```python
from build123d import *

# Parameters (mm, degrees)
BOSS_EXTRUDE1_DEPTH      = 40
CUT_EXTRUDE1_DEPTH       = 45
CUT_EXTRUDE2_REACH       = 47.222
SKETCH3_W                = 12
SKETCH3_H                = 10
SKETCH4_R                = 2.55
CUT_EXTRUDE3_DEPTH       = 17.5
FILLET4_R                = 2
CUT_EXTRUDE5_START       = -12.324555
SKETCH6_R                = 2.5
CUT_EXTRUDE5_DEPTH       = 9.6
CUT_EXTRUDE6_START       = 6.279445
SKETCH6_3_R              = 2.5
CUT_EXTRUDE6_DEPTH       = 6.604
CUT_EXTRUDE7_START       = -14.986
CUT_EXTRUDE7_DEPTH       = 14.986
CUT_EXTRUDE14_DEPTH      = 10
CUT_EXTRUDE14_DEPTH_BACK = 20
FILLET3_R                = 1
CUT_EXTRUDE17_DEPTH      = 9
CUT_EXTRUDE17_DEPTH_BACK = 31
SKETCH19_W               = 34.391960709
SKETCH19_H               = 80.468832088
SKETCH20_R               = 3.25
BOSS_EXTRUDE2_DEPTH      = 2
SKETCH21_R               = 1.5
CUT_EXTRUDE18_DEPTH      = 14
CUT_EXTRUDE19_START      = -4
SKETCH22_R               = 2.5
CUT_EXTRUDE19_DEPTH      = 14
CUT_EXTRUDE20_DEPTH      = 14
CUT_EXTRUDE20_DEPTH_BACK = 14


with BuildPart() as part:
    # Sketch1 → Boss-Extrude1 (new body)
    with BuildSketch(Plane(origin=(0, 0, 0), x_dir=(1, 0, 0), z_dir=(0, 1, 0))):
        with BuildLine():
            Line((-6.32455532, 9), (6.32455532, 9))
            ThreePointArc((6.32455532, 9), (11, 0), (6.32455532, -9))
            Line((6.32455532, -9), (-6.32455532, -9))
            ThreePointArc((-6.32455532, -9), (-11, 0), (-6.32455532, 9))
        make_face()
    extrude(amount=BOSS_EXTRUDE1_DEPTH)

    # Sketch2 → Cut-Extrude1 (cut)
    with BuildSketch(Plane.XZ):
        with BuildLine():
            Line((1.5, 5), (-1.5, 5))
            ThreePointArc((-1.5, 5), (0, 6.5), (1.5, 5))
        make_face()
        with BuildLine():
            Line((1.5, -5), (-1.5, -5))
            ThreePointArc((-1.5, -5), (0, -6.5), (1.5, -5))
        make_face()
    extrude(amount=-CUT_EXTRUDE1_DEPTH, mode=Mode.SUBTRACT)

    # Cut-Extrude2: up to this face of the body (flat: up to its plane)
    cut_extrude2_end = Plane(part.part.faces().sort_by_distance((0, 20, 9))[0])
    # Sketch3 → Cut-Extrude2 (cut, up to the picked face)
    with BuildSketch(Plane(origin=(0, 0, -9), x_dir=(-1, 0, 0), z_dir=(0, 0, -1)), mode=Mode.PRIVATE) as cut_extrude2_sk1:
        with Locations((0, 5)):
            Rectangle(SKETCH3_W, SKETCH3_H)
    cut_extrude2_tool1 = split(extrude(cut_extrude2_sk1.sketch, amount=-CUT_EXTRUDE2_REACH, mode=Mode.PRIVATE), bisect_by=cut_extrude2_end, keep=Keep.BOTH, mode=Mode.PRIVATE)
    add(cut_extrude2_tool1.solids().sort_by(Axis((0, 5, -9), (0, 0, 1)))[0], mode=Mode.SUBTRACT)

    # Sketch4 → Cut-Extrude3 (cut, symmetric)
    with BuildSketch(Plane.ZY.offset(-6)):
        with Locations(Location((0, 4.9, 0), (0, 0, 270))):
            Circle(SKETCH4_R)
        with BuildLine():
            Line((-9, 10), (-4.9, 4.9))
            ThreePointArc((-4.9, 4.9), (0, 0), (4.9, 4.9))
            Line((4.9, 4.9), (9, 10))
            Line((9, 10), (12.043777938, -1.930413563))
            Line((12.043777938, -1.930413563), (-10.290438773, -1.930413563))
            Line((-10.290438773, -1.930413563), (-9, 10))
        make_face()
    extrude(amount=CUT_EXTRUDE3_DEPTH, both=True, mode=Mode.SUBTRACT)

    # Fillet4
    fillet4_edges = [part.edges().sort_by_distance(p)[0] for p in [
        (0, 10, 5),
        (0, 10, 6.5),
        (0, 10, -5),
        (0, 10, -6.5),
    ]]
    fillet(fillet4_edges, radius=FILLET4_R)

    # Sketch6 → Cut-Extrude5 (cut)
    with BuildSketch(Plane.ZY.offset(6.32455532).offset(CUT_EXTRUDE5_START)):
        with BuildLine():
            Line((9, 22.232353468), (0, 30))
            ThreePointArc((0, 30), (-3.535533906, 31.464466094), (-5, 35))
            Line((-5, 35), (-6.715621335, 37.134065563))
            ThreePointArc((-6.715621335, 37.134065563), (-7.737273484, 38.043034193), (-9, 38.567933069))
            Line((-9, 38.567933069), (-20.985236203, 70.297327945))
            Line((-20.985236203, 70.297327945), (29.827478779, 37.594689174))
            Line((29.827478779, 37.594689174), (9, 22.232353468))
        make_face()
        with Locations((0, 35)):
            Circle(SKETCH6_R, mode=Mode.SUBTRACT)
    extrude(amount=-CUT_EXTRUDE5_DEPTH, mode=Mode.SUBTRACT)

    # Sketch6<3> → Cut-Extrude6 (cut)
    with BuildSketch(Plane.ZY.offset(6.32455532).offset(CUT_EXTRUDE6_START)):
        with BuildLine():
            Line((9, 22.232353468), (0, 30))
            ThreePointArc((0, 30), (-3.535533906, 31.464466094), (-5, 35))
            Line((-5, 35), (-6.715621335, 37.134065563))
            ThreePointArc((-6.715621335, 37.134065563), (-7.737273484, 38.043034193), (-9, 38.567933069))
            Line((-9, 38.567933069), (-20.985236203, 70.297327945))
            Line((-20.985236203, 70.297327945), (29.827478779, 37.594689174))
            Line((29.827478779, 37.594689174), (9, 22.232353468))
        make_face()
        with Locations((0, 35)):
            Circle(SKETCH6_3_R, mode=Mode.SUBTRACT)
    extrude(amount=-CUT_EXTRUDE6_DEPTH, mode=Mode.SUBTRACT)

    # Sketch7 → Cut-Extrude7 (cut)
    with BuildSketch(Plane(origin=(6, 0, 0), x_dir=(0, 0, -1), z_dir=(1, 0, 0)).offset(CUT_EXTRUDE7_START)):
        with BuildLine():
            Line((5, 35), (6.715621335, 37.134065563))
            ThreePointArc((6.715621335, 37.134065563), (7.737273484, 38.043034193), (9, 38.567933069))
            Line((9, 38.567933069), (17.905522107, 46.18977372))
            Line((17.905522107, 46.18977372), (-20.628346566, 40.15215478))
            Line((-20.628346566, 40.15215478), (-9, 22.232353468))
            Line((-9, 22.232353468), (-5, 25.684640815))
            Line((-5, 25.684640815), (-5, 35))
            ThreePointArc((-5, 35), (0, 40), (5, 35))
        make_face()
    extrude(amount=CUT_EXTRUDE7_DEPTH, mode=Mode.SUBTRACT)

    # Sketch16 → Cut-Extrude14 (cut, two sides: drawn at the far end of the back side and taken through both)
    with BuildSketch(Plane.ZY.offset(6.32455532).offset(-CUT_EXTRUDE14_DEPTH_BACK)):
        Polygon((8.113259987, 8.896981935), (11.550119513, 20.031417135), (18.056002312, 15.695207893), (16.156055326, 2.281594324), align=None)
    extrude(amount=CUT_EXTRUDE14_DEPTH + CUT_EXTRUDE14_DEPTH_BACK, mode=Mode.SUBTRACT)

    # Fillet3
    # the kernel refuses this fillet: 1 mm, written as the material it takes off along each edge
    with BuildSketch(Plane(origin=(5.99999968, 23.184640014, 5), x_dir=(-1, 0, 0), z_dir=(0, 1, 0))) as fillet3_piece_1_section:
        with BuildLine():
            CenterArc((FILLET3_R, -FILLET3_R), FILLET3_R, 90, 90)
            Line((0, -FILLET3_R), (0, 0))
            Line((0, 0), (FILLET3_R, 0))
        make_face()
    fillet3_piece_1 = extrude(amount=11.815359986, mode=Mode.PRIVATE)
    fillet3_piece_1 = split(fillet3_piece_1, bisect_by=Plane(origin=(5.764976342, 27.542151825, 2.84779096), z_dir=(0, 0.7570343753275036, 0.6533750489362878)), keep=Keep.TOP, mode=Mode.PRIVATE)
    add(fillet3_piece_1, mode=Mode.SUBTRACT)
    with BuildSketch(Plane(origin=(6, 35, 0), x_dir=(0, 0, 1), z_dir=(0, -1, 0))) as fillet3_piece_2_section:
        with BuildLine():
            CenterArc((4, 1.00000032), FILLET3_R, 270, 90)
            ThreePointArc((4, 3.2e-07), (4.5, 3.2e-07), (5, 0))
            Line((5, 0), (5, 1.00000032))
        make_face()
    fillet3_piece_2 = revolve(axis=Axis((6, 35, 0), (-1, 0, 0)), revolution_arc=208.693968336, mode=Mode.PRIVATE)
    fillet3_piece_2 = split(fillet3_piece_2, bisect_by=Plane(origin=(5.717618036, 35.865387036, -5.695703303), z_dir=(0, 0.6265569118246621, 0.7793756708062823)), keep=Keep.TOP, mode=Mode.PRIVATE)
    add(fillet3_piece_2, mode=Mode.SUBTRACT)
    with BuildSketch(Plane(origin=(-6.00000032, 35, 0), x_dir=(0, -0.48013104288571345, -0.8771967747646346), z_dir=(0, -0.8771967747646346, 0.48013104288571345))) as fillet3_piece_3_section:
        with BuildLine():
            CenterArc((5 - FILLET3_R, FILLET3_R), FILLET3_R, 270, 90)
            Line((5 - FILLET3_R, 0), (5, 0))
            Line((5, 0), (5, FILLET3_R))
        make_face()
    fillet3_piece_3 = revolve(axis=Axis((-6.00000032, 35, 0), (1, 0, 0)), revolution_arc=208.69396098, mode=Mode.PRIVATE)
    fillet3_piece_3 = split(fillet3_piece_3, bisect_by=Plane(origin=(-5.717618693, 35.865387047, -5.695703312), z_dir=(0, 0.6265569118246621, 0.7793756708062823)), keep=Keep.TOP, mode=Mode.PRIVATE)
    add(fillet3_piece_3, mode=Mode.SUBTRACT)
    with BuildSketch(Plane(origin=(-6.00000032, 35, 5), x_dir=(0, 0, -1), z_dir=(0, -1, 0))) as fillet3_piece_4_section:
        with BuildLine():
            CenterArc((FILLET3_R, FILLET3_R), FILLET3_R, 180, 90)
            Line((0, FILLET3_R), (0, 0))
            Line((0, 0), (FILLET3_R, 0))
        make_face()
    fillet3_piece_4 = extrude(amount=11.815359185, mode=Mode.PRIVATE)
    fillet3_piece_4 = split(fillet3_piece_4, bisect_by=Plane(origin=(-5.831638788, 29.468233541, 0.616132326), z_dir=(0, 0.7570343753275036, 0.6533750489362878)), keep=Keep.TOP, mode=Mode.PRIVATE)
    add(fillet3_piece_4, mode=Mode.SUBTRACT)

    # Sketch19 → Cut-Extrude17 (cut, two sides: drawn at the far end of the back side and taken through both)
    with BuildSketch(Plane.XY.offset(5).offset(-CUT_EXTRUDE17_DEPTH_BACK)):
        with Locations((-13.695980355, 34.702359308)):
            Rectangle(SKETCH19_W, SKETCH19_H)
    extrude(amount=CUT_EXTRUDE17_DEPTH + CUT_EXTRUDE17_DEPTH_BACK, mode=Mode.SUBTRACT)

    # Sketch20 → Boss-Extrude2 (add)
    with BuildSketch(Plane.ZY.offset(-3.5)):
        with Locations(Location((0, 20.3, 0), (0, 0, 270))):
            Circle(SKETCH20_R)
    extrude(amount=BOSS_EXTRUDE2_DEPTH)

    # Sketch21 → Cut-Extrude18 (cut)
    with BuildSketch(Plane.ZY.offset(-1.5)):
        with Locations(Location((0, 20.3, 0), (0, 0, 270))):
            Circle(SKETCH21_R)
    extrude(amount=-CUT_EXTRUDE18_DEPTH, mode=Mode.SUBTRACT)

    # Sketch22 → Cut-Extrude19 (cut)
    with BuildSketch(Plane.ZY.offset(-1.5).offset(CUT_EXTRUDE19_START)):
        with Locations(Location((0, 20.3, 0), (0, 0, 270))):
            Circle(SKETCH22_R)
    extrude(amount=-CUT_EXTRUDE19_DEPTH, mode=Mode.SUBTRACT)

    # Sketch17 → Cut-Extrude20 (cut, two sides: drawn at the far end of the back side and taken through both)
    with BuildSketch(Plane.XY.offset(-CUT_EXTRUDE20_DEPTH_BACK)):
        with BuildLine():
            Line((11, 0), (25.575472319, 70.054686952))
            Line((25.575472319, 70.054686952), (-19.116979593, 73.080460091))
            Line((-19.116979593, 73.080460091), (-22.103338511, 10.056999989))
            Line((-22.103338511, 10.056999989), (-11, 0))
            ThreePointArc((-11, 0), (-9.292734081, 20), (-11, 40))
            Line((-11, 40), (-11, 54.709335657))
            Line((-11, 54.709335657), (1.039161205, 61.782229983))
            Line((1.039161205, 61.782229983), (17.277292868, 53.927851901))
            Line((17.277292868, 53.927851901), (11, 40))
            ThreePointArc((11, 40), (9.292734081, 20), (11, 0))
        make_face()
    extrude(amount=CUT_EXTRUDE20_DEPTH + CUT_EXTRUDE20_DEPTH_BACK, mode=Mode.SUBTRACT)


solid = part.part
```
The model under review builds one solid part; all positions refer to its coordinate system, in mm. A direction names the side the tool comes from. Give positions to 0.01 mm unless a question says otherwise; leave off trailing zeros. Write each loop counter-clockwise with the first axis right and the second up, starting at its lowest first coordinate (ties: lowest second). Pieces come first, ordered by that corner, then holes. Notation, with made-up numbers: M 40,26.25 L 65,26.25 A22 ccw 65,64.25 Z; hole C 47,73.5 d10. An arc over 180 degrees is marked long. Write item = value, one per line. Start each with the question number.
Q1. Machinability: for faces 1 (the face through (8.27, 37.11, 1.34)), 2 (the face through (5.699, 30.277, 4.715)), 3 (the face through (5, 10, 0)), which of the approach directions +Z, -Z, +X, -X, +Y, -Y give a long, thin tool a straight path to every point of the face, cutting with its end or side? Answer none if there is none.
Q2. Clearance check with flat-ended pins moving along their axes: pin 1 (7 mm diameter, centred on y = 35.5, z = -2, fed in from +X); pin 2 (2.5 mm diameter, centred on y = 20, z = -0.5, fed in from +X); pin 3 (1.6 mm diameter, centred on x = 4.5, y = 30, fed in from +Z). State where each tip first meets the part, or that it passes through.
Q3. We need section A-A (x = 4). State the section outline as (y, z) points.
Q4. For line 1 (Y direction, x = 8.7, z = 0); line 2 (Z direction, x = 2.85, y = 20.3); line 3 (Z direction, x = 9.15, y = 4.9), list the stretches that pass through material, from the lowest coordinate up.
Q5. We need section B-B (y = 20.3). State the section outline as (x, z) points, plus the area to 3 significant figures.
Q6. Mouldability with a two-part tool opening along Z and no side actions: class faces 4 (the face through (1.5, 22, -1)), 5 (the face through (8.28, 2.47, 0.77)), 6 (the face through (2.514, 23.547, 0.143)) as released by +Z, released by -Z, zero draft, split by the parting line, or undercut.
Result set:
q1.face_1 = +X
q1.face_2 = +Z, +X, +Y
q1.face_3 = +Z, -Z, -X, -Y
q2.pin_1 = 10.6
q2.pin_2 = 5.5
q2.pin_3 = 5
q3.outline = M 10,-9 L 38.57,-9 A4.12 ccw 37.13,-6.72 L 35,-5 A5 ccw 35,5 L 25.68,5 L 22.23,9 L 11.77,9 L 10,8.45 Z; hole C 20.3,0 d3
q4.line_1 = 0 to 2.35, 7.45 to 17.8, 22.8 to 30, 32.5 to 37.5
q4.line_2 = -3.25 to -1.5, 1.5 to 3.25
q4.line_3 = -4.9 to -2.55, 2.55 to 4.9
q5.outline = M 1.5,-3.25 L 3.5,-3.25 L 3.5,-9 L 6.32,-9 A11 ccw 9.29,-5.89 L 9.29,-2.5 L 5.5,-2.5 L 5.5,-1.5 L 1.5,-1.5 Z; M 1.5,1.5 L 5.5,1.5 L 5.5,2.5 L 9.29,2.5 L 9.29,5.89 A11 ccw 6.32,9 L 3.5,9 L 3.5,3.25 L 1.5,3.25 Z
q5.area = 78.3 mm2
q6.face_4 = zero draft
q6.face_5 = undercut
q6.face_6 = split by the parting line
